Input: part model. Units: mm. Frame: model coordinates. Give positions to 0.01 mm unless a question says otherwise; leave off trailing zeros. Loops run counter-clockwise (first coordinate to the right, second up) from the corner with the lowest first, then second, coordinate; pieces in that order, holes last.
from build123d import *

# Parameters (mm, degrees)
F0_W     = 12.7
F0_H     = 90.8
F0_W_2   = 59.05
F0_R     = 2.921
F1_DEPTH = 12.7
F2_DEPTH = 190.5


with BuildPart() as f1:
    # F0 (on Top) → F1 (new body)
    with BuildSketch(Plane.XY):
        with Locations((39.05, 0)):
            Rectangle(F0_W, F0_H)
        with Locations((3.175, 0)):
            Rectangle(F0_W_2, F0_H)
        with Locations((-14.142136, -14.142136)):
            Circle(F0_R, mode=Mode.SUBTRACT)
        with Locations((14.142136, -14.142136)):
            Circle(F0_R, mode=Mode.SUBTRACT)
        with Locations((-14.142136, 14.142136)):
            Circle(F0_R, mode=Mode.SUBTRACT)
        with Locations((14.142136, 14.142136)):
            Circle(F0_R, mode=Mode.SUBTRACT)
    extrude(amount=F1_DEPTH)

    # F0 (on Top) → F2 (join)
    with BuildSketch(Plane.XY):
        with Locations((39.05, 0)):
            Rectangle(F0_W, F0_H)
    extrude(amount=F2_DEPTH)


with BuildPart() as f3_1:
    # F3: copy of F1
    add(f1.part)


solid = f1.part
(1) Mould query, pull axis X, two halves, no side actions, for faces 1 (the cylindrical face through (13.762, -11.246, 6.261)), 2 (the flat face through (3, 1, 12.7)), 3 (the flat face through (32.7, -1, 100)), 4 (the flat face through (45.4, -1, 94)). Classes: +X half, -X half, draft (parallel to the pull), parting line (faces both ways), or undercut.
Values follow:
face 1: undercut
face 2: draft
face 3: -X half
face 4: +X half
(2) Cut plane D-D (z = 41). Return the cut outline in (x, y).
Values follow:
outline: (32.7, -45.4) - (45.4, -45.4) - (45.4, 45.4) - (32.7, 45.4) - close
(3) Ray query, probe 1 along Z at (x, y) = (-10, -12); probe 2 along X at (y, z) = (29, 48). Return the intervals inside material, ascending.
Values follow:
probe 1: z = 0 to 12.7
probe 2: x = 32.7 to 45.4
(4) Cut plane B-B (y = -39.5). Return the cut outline in (x, z), and give its area (3 significant figures).
Values follow:
outline: (-26.35, 0) - (45.4, 0) - (45.4, 190.5) - (32.7, 190.5) - (32.7, 12.7) - (-26.35, 12.7) - close
area: 3,170 mm2
(5) Pin query (flat end, axial travel): pin 1 Ø6 at (x, y) = (10.5, -21) entering from +Z; pin 2 Ø7.5 at (x, y) = (-14.14, -14.14) entering from -Z; pin 3 Ø4.5 at (x, y) = (14.14, 14.14) entering from +Z; pin 4 Ø2 at (y, z) = (5, 27.5) entering from -X. Return the tip coordinate at first contact, or that it passes through.
Values follow:
pin 1: stops at z = 12.7
pin 2: stops at z = 0
pin 3: passes through
pin 4: stops at x = 32.7
(6) Cut plane C-C (x = -5). Return the cut outline in (y, z), and give its area (3 significant figures).
Values follow:
outline: (-45.4, 0) - (45.4, 0) - (45.4, 12.7) - (-45.4, 12.7) - close
area: 1,150 mm2
(7) Cut plane A-A (x = -15). Return the cut outline in (y, z), and give its area (3 significant figures).
Values follow:
outline: (-45.4, 0) - (-16.93, 0) - (-16.93, 12.7) - (-45.4, 12.7) - close; (-11.35, 0) - (11.35, 0) - (11.35, 12.7) - (-11.35, 12.7) - close; (16.93, 0) - (45.4, 0) - (45.4, 12.7) - (16.93, 12.7) - close
area: 1,010 mm2
